Can you work these out from the model? Positions are in its coordinate system, mm. A direction names the side the tool comes from. Give positions to 0.01 mm unless a question says otherwise; leave off trailing zeros. Loops run counter-clockwise (first coordinate to the right, second up) from the corner with the lowest first, then second, coordinate; pieces in that order, holes last. Notation, with made-up numbers: M 75.5,-23.5 L 109.5,-23.5 A20 ccw 109.5,9.5 Z; hole C 79.5,-24.5 d5. An arc over 180 degrees is marked long. Put each result on its own line as item: value. Start each with the question number.
1) Imagine slicing it at A-A (x = -80). Write out the boundary of the cut face in (y, z).
2) For P1, Ø6, axis at y = -56, z = 943, coming from the +X side; P2, Ø1.5, axis at x = -96, z = 986, coming from the -Y side; P3, Ø8, axis at y = -113.5, z = 776.5, coming from the +X side; P4, Ø1, axis at x = -19.5, y = 38.5, coming from the -Z side, each with a flat end and sliding along its axis, tell me the tip position at first contact or that it passes through.
3) Please list where these lines run through material, in increasing order: line 1 along Z through (x, y) = (42.5, 98.5); line 2 along X through (y, z) = (-28.5, 723). Write a range as from..to.
4) For faces 1 (the flat face through (-59, -110, 635)), 2 (the flat face through (-120, -64, 635)), 3 (the flat face through (-2, 2, 0)), 4 (the flat face through (-66, -120, 635)), which set-ups out of +Z, -Z, +X, -X, +Y, -Y let a thin tool reach every point of the face, with its end or its side?
5) Imagine slicing it at C-C (z = 380.5). Write out the boundary of the cut face in (x, y).
6) Imagine slicing it at D-D (x = 45). Write out the boundary of the cut face in (y, z).
from build123d import *

# Parameters (mm, degrees)
F0_W     = 250
F0_H     = 250
F1_DEPTH = 15
F3_DEPTH = 1257


with BuildPart() as f1:
    # F0 (on Top) → F1 (new body)
    with BuildSketch(Plane.XY):
        Rectangle(F0_W, F0_H)
    extrude(amount=F1_DEPTH)

    # F2 (on face) → F3 (join)
    with BuildSketch(Plane.XY.offset(15)):
        Polygon((-110, -10), (-120, -10), (-120, -110), (-120, -120), (-110, -120), (-10, -120), (-10, -110), (-110, -110), align=None)
    extrude(amount=F3_DEPTH)


solid = f1.part
Recorded:
1. outline: M -125,0 L 125,0 L 125,15 L -110,15 L -110,1272 L -120,1272 L -120,15 L -125,15 Z
2. P1: x = -110
2. P2: y = -120
2. P3: x = -10
2. P4: z = 0
3. line 1: 0..15
3. line 2: -120..-110
4. face 1: +Z, +X, +Y
4. face 2: +Z, -X, +Y, -Y
4. face 3: -Z, +X, -X, +Y, -Y
4. face 4: +Z, +X, -X, -Y
5. outline: M -120,-120 L -10,-120 L -10,-110 L -110,-110 L -110,-10 L -120,-10 Z
6. outline: M -125,0 L 125,0 L 125,15 L -125,15 Z
